from build123d import *

# Parameters (mm, degrees)
BOX002_W     = 0.75
BOX002_H     = 25
BOX002_DEPTH = 10
BOX003_W     = 0.75
BOX003_H     = 25
BOX003_DEPTH = 10
BOX004_W     = 0.75
BOX004_H     = 25
BOX004_DEPTH = 10
BOX001_W     = 0.75
BOX001_H     = 25
BOX001_DEPTH = 10
BOX_W        = 22
BOX_H        = 35
BOX_DEPTH    = 5
FILLET_R     = 4


with BuildPart() as cube002:
    # Box002 → Box002 (new body)
    with BuildSketch(Plane(origin=(11.5, 5, 0), x_dir=(1, 0, 0), z_dir=(0, 0, 1))):
        with Locations((0.375, 12.5)):
            Rectangle(BOX002_W, BOX002_H)
    extrude(amount=BOX002_DEPTH)


with BuildPart() as cube003:
    # Box003 → Box003 (new body)
    with BuildSketch(Plane(origin=(7.75, 5, 0), x_dir=(1, 0, 0), z_dir=(0, 0, 1))):
        with Locations((0.375, 12.5)):
            Rectangle(BOX003_W, BOX003_H)
    extrude(amount=BOX003_DEPTH)


with BuildPart() as cube004:
    # Box004 → Box004 (new body)
    with BuildSketch(Plane(origin=(16.25, 5, 0), x_dir=(1, 0, 0), z_dir=(0, 0, 1))):
        with Locations((0.375, 12.5)):
            Rectangle(BOX004_W, BOX004_H)
    extrude(amount=BOX004_DEPTH)


with BuildPart() as fusion:
    # Box001 → Box001 (new body)
    with BuildSketch(Plane(origin=(5, 5, 0), x_dir=(1, 0, 0), z_dir=(0, 0, 1))):
        with Locations((0.375, 12.5)):
            Rectangle(BOX001_W, BOX001_H)
    extrude(amount=BOX001_DEPTH)

    # Fusion: union Cube002, Cube003, Cube004
    add(cube002.part)
    add(cube003.part)
    add(cube004.part)


with BuildPart() as cut:
    # Box → Box (new body)
    with BuildSketch(Plane.XY):
        with Locations((11, 17.5)):
            Rectangle(BOX_W, BOX_H)
    extrude(amount=BOX_DEPTH)

    # Fillet
    fillet_edges = [cut.edges().sort_by_distance(p)[0] for p in [
        (0, 0, 2.5),
        (0, 35, 2.5),
        (22, 0, 2.5),
        (22, 35, 2.5),
    ]]
    fillet(fillet_edges, radius=FILLET_R)

    # Cut: cut Fusion
    add(fusion.part, mode=Mode.SUBTRACT)


solid = cut.part
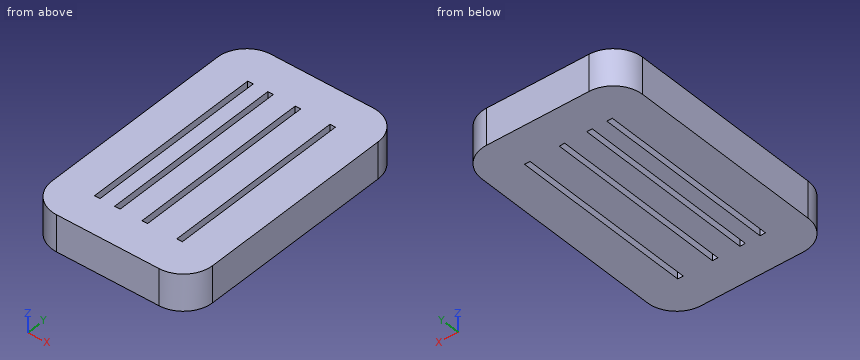
Could you check a few things on this model? Use its own coordinates, in mm. Give positions to 0.01 mm unless a question says otherwise; leave off trailing zeros. Loops run counter-clockwise (first coordinate to the right, second up) from the corner with the lowest first, then second, coordinate; pieces in that order, holes last. Notation, with made-up numbers: (55, -1.5) -> (69, -1.5) arc R13 cw to (69, 13.5) -> close; hole circle Ø5 at (-34.5, 15). An arc over 180 degrees is marked (long way). Return JSON: item names as keys, results as strings.
Item 1: If we section it at C-C on x = 19.5: List the corners of the cut face in (y, z) for me.
Geometry results:
{"outline": "(0.29, 0) -> (34.71, 0) -> (34.71, 5) -> (0.29, 5) -> close"}
Item 2: If we section it at D-D on x = 1.5: List the corners of the cut face in (y, z) for me.
Geometry results:
{"outline": "(0.88, 0) -> (34.12, 0) -> (34.12, 5) -> (0.88, 5) -> close"}
Item 3: I'm going to push a flat-ended pin straight in: pin 1 (4 mm diameter, centred on x = 16, y = 7.5, fed in from -Z). Where does the tip first touch, or does it pass through?
Geometry results:
{"pin 1": "stops at z = 0"}
Item 4: If we section it at B-B on z = 0.7: List the corners of the cut face in (x, y) for me, plus the area to 3 significant figures.
Geometry results:
{"outline": "(0, 4) arc R4 ccw to (4, 0) -> (18, 0) arc R4 ccw to (22, 4) -> (22, 31) arc R4 ccw to (18, 35) -> (4, 35) arc R4 ccw to (0, 31) -> close; hole (5, 5) -> (5.75, 5) -> (5.75, 30) -> (5, 30) -> close; hole (7.75, 5) -> (8.5, 5) -> (8.5, 30) -> (7.75, 30) -> close; hole (11.5, 5) -> (12.25, 5) -> (12.25, 30) -> (11.5, 30) -> close; hole (16.25, 5) -> (17, 5) -> (17, 30) -> (16.25, 30) -> close", "area": "681 mm²"}
Item 5: If we section it at A-A on y = 24: List the corners of the cut face in (x, z) for me.
Geometry results:
{"outline": "(0, 0) -> (5, 0) -> (5, 5) -> (0, 5) -> close; (5.75, 0) -> (7.75, 0) -> (7.75, 5) -> (5.75, 5) -> close; (8.5, 0) -> (11.5, 0) -> (11.5, 5) -> (8.5, 5) -> close; (12.25, 0) -> (16.25, 0) -> (16.25, 5) -> (12.25, 5) -> close; (17, 0) -> (22, 0) -> (22, 5) -> (17, 5) -> close"}
Item 6: I need wall thicknesses on L1, parallel to X at y = 11, z = 1.85; L2, parallel to Y at x = 5.25, z = 4.4; L3, parallel to Y at x = 2.25, z = 0.3. Which ranges of each line are inside material? Lowest first, please. Write a range as from..to.
Geometry results:
{"L1": "x = 0..5, 5.75..7.75, 8.5..11.5, 12.25..16.25, 17..22", "L2": "y = 0..5, 30..35", "L3": "y = 0.4..34.6"}
